Design review of the part built by this model. Coordinates are the model's own, in mm. Face numbers are marked on the shaded views. Coordinates: 2 decimals unless noted, no trailing zeros. Write each loop counter-clockwise with the first axis right and the second up, starting at its lowest first coordinate (ties: lowest second). Pieces come first, ordered by that corner, then holes. Notation, with made-up numbers: (13.5, 89.25) -> (70.5, 89.25) arc R27 ccw to (70.5, 112.25) -> close; hole circle Ø7 at (78.25, 85). An arc over 180 degrees is marked (long way). Answer in a Markdown table with one row per item. Add a question column.
Item 1: Take a section at B-B, the plane x = 0. Write out the cut boundary in (y, z), and give its area (3 significant figures).
Item 2: Clearance check with flat-ended pins moving along their axes: P1, Ø3, axis at y = 3.5, z = 9, coming from the +X side; P2, Ø8, axis at x = -5, z = -10.5, coming from the -Y side; P3, Ø5, axis at y = 4.5, z = -3.5, coming from the +X side; P4, Ø1, axis at x = -4, z = -6.5, coming from the +Y side. State where each tip first meets the part, or that it passes through.
Item 3: Draft analysis for pull direction X (two halves, no side actions). For the marked faces 1, 2 and 3, state which applies: released by +X, released by -X, zero draft, split by the parting line, or undercut.
Item 4: Take a section at D-D, the plane x = -13. Write out the cut boundary in (y, z).
Item 5: To check wall thickness, follow line 1 (X direction, y = 9, z = 0); line 2 (X direction, y = 3, z = -0.25); line 3 (Y direction, x = -2.75, z = 9.5). State the ranges of each line that lie inside material, in increasing order.
Item 6: Take a section at C-C, the plane z = 13. Write out the cut boundary in (x, y), and give its area (3 significant figures).
Item 7: Take a section at A-A, the plane y = 18.25. Write out the cut boundary in (x, z).
from build123d import *

# Parameters (mm, degrees)
SKETCH1_R                = 15
BOSS_EXTRUDE1_DEPTH      = 4
SKETCH2_R                = 15
SKETCH2_R_2              = 11
BOSS_EXTRUDE2_DEPTH      = 15
SKETCH3_R                = 0.9
BOSS_EXTRUDE3_DEPTH      = 3
FILLET1_R                = 0.5
CIRPATTERN1_COUNT        = 4
FILLET1_OF_CIRPATTERN1_R = 0.5
FILLET2_R                = 1


with BuildPart() as part:
    # Sketch1 → Boss-Extrude1 (new body)
    with BuildSketch(Plane(origin=(0, 0, 0), x_dir=(1, 0, 0), z_dir=(0, 1, 0))):
        with Locations(Location((0, 0, 0), (0, 0, 270))):
            Circle(SKETCH1_R)
    extrude(amount=BOSS_EXTRUDE1_DEPTH)

    # Sketch2 → Boss-Extrude2 (add)
    with BuildSketch(Plane(origin=(0, 4, 0), x_dir=(1, 0, 0), z_dir=(0, 1, 0))):
        with Locations(Location((0, 0, 0), (0, 0, 270))):
            Circle(SKETCH2_R)
        with Locations(Location((0, 0, 0), (0, 0, 270))):
            Circle(SKETCH2_R_2, mode=Mode.SUBTRACT)
    extrude(amount=BOSS_EXTRUDE2_DEPTH)

    # Sketch3 → Boss-Extrude3 (add)
    with BuildSketch(Plane(origin=(0, 19, 0), x_dir=(1, 0, 0), z_dir=(0, 1, 0))):
        with Locations(Location((0, -13, 0), (0, 0, 270))):
            Circle(SKETCH3_R)
    boss_extrude3 = extrude(amount=BOSS_EXTRUDE3_DEPTH)

    # Fillet1
    fillet1_edges = [part.edges().sort_by_distance(p)[0] for p in [
        (0, 19, 12.1),
    ]]
    fillet(fillet1_edges, radius=FILLET1_R)

    # CirPattern1: Boss-Extrude3 ×4 about axis
    cirpattern1_axis = Axis((0, 0, 0), (0, 1, 0))
    for i in range(1, CIRPATTERN1_COUNT):
        add(boss_extrude3.rotate(cirpattern1_axis, i * 360 / CIRPATTERN1_COUNT))

    # Fillet1 of CirPattern1
    fillet1_of_cirpattern1_edges = [part.edges().sort_by_distance(p)[0] for p in [
        (12.1, 19, 0),
        (0, 19, -12.1),
        (-12.1, 19, 0),
    ]]
    fillet(fillet1_of_cirpattern1_edges, radius=FILLET1_OF_CIRPATTERN1_R)

    # Fillet2
    fillet2_edges = [part.edges().sort_by_distance(p)[0] for p in [
        (0, 4, -11),
    ]]
    fillet(fillet2_edges, radius=FILLET2_R)


solid = part.part
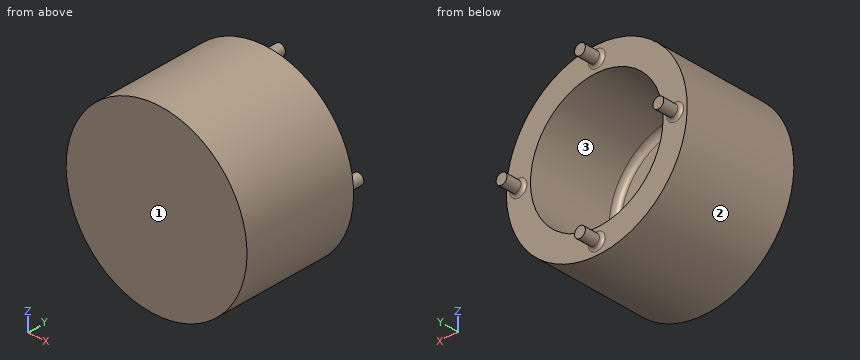
Answers:
| question | item | result |
|---|---|---|
| 1 | outline | (0, -15) -> (19, -15) -> (19, -14.4) arc R0.5 cw to (19.5, -13.9) -> (22, -13.9) -> (22, -12.1) -> (19.5, -12.1) arc R0.5 cw to (19, -11.6) -> (19, -11) -> (5, -11) arc R1 cw to (4, -10) -> (4, 10) arc R1 cw to (5, 11) -> (19, 11) -> (19, 11.6) arc R0.5 cw to (19.5, 12.1) -> (22, 12.1) -> (22, 13.9) -> (19.5, 13.9) arc R0.5 cw to (19, 14.4) -> (19, 15) -> (0, 15) -> close |
| 1 | area | 251 mm^2 |
| 2 | P1 | stops at x = 12.99 |
| 2 | P2 | stops at y = 0 |
| 2 | P3 | stops at x = 14.97 |
| 2 | P4 | stops at y = 4 |
| 3 | face 1 | zero draft |
| 3 | face 2 | split by the parting line |
| 3 | face 3 | undercut |
| 4 | outline | (0, -7.48) -> (19, -7.48) -> (19, -1.4) arc R0.5 cw to (19.5, -0.9) -> (22, -0.9) -> (22, 0.9) -> (19.5, 0.9) arc R0.5 cw to (19, 1.4) -> (19, 7.48) -> (0, 7.48) -> close |
| 5 | line 1 | x = -15 to -11, 11 to 15 |
| 5 | line 2 | x = -15 to 15 |
| 5 | line 3 | y = 0 to 4 |
| 6 | outline | (-7.48, 0) -> (7.48, 0) -> (7.48, 19) -> (1.4, 19) arc R0.5 cw to (0.9, 19.5) -> (0.9, 22) -> (-0.9, 22) -> (-0.9, 19.5) arc R0.5 cw to (-1.4, 19) -> (-7.48, 19) -> close |
| 6 | area | 290 mm^2 |
| 7 | outline | circle Ø30 at (0, 0); hole circle Ø22 at (0, 0) |
